Build history of the part. All positions in model axes, mm. Coordinates: 2 decimals unless noted, no trailing zeros. Order: outer loops, then holes, each group sorted by start corner. A loop starts at its lowest first (then second) coordinate and runs counter-clockwise, first axis right, second up. Notation, with made-up numbers: (-35, 22) - (-8, 22) arc R27 ccw to (-8, 54) - close; hole circle Ø10 at (-37.5, 61.25). An arc over 180 degrees is marked (long way). Write each question's results on one line, items separated by ' | '.
from build123d import *

# Parameters (mm, degrees)
SKETCH_1_W          = 38
SKETCH_1_H          = 35
EXTRUDE_1_DEPTH     = 5
CHAMFER_1_SIZE      = 0.5
SKETCH_2_R          = 2.25
SKETCH_2_R_2        = 2
CUT_EXTRUDE_1_DEPTH = 52.903757089


with BuildPart() as part:
    # 草图1 → 凸台-拉伸1 (new body)
    with BuildSketch(Plane(origin=(0, 0, 0), x_dir=(1, 0, 0), z_dir=(0, 1, 0))):
        with Locations((19, 17.5)):
            Rectangle(SKETCH_1_W, SKETCH_1_H)
    extrude(amount=EXTRUDE_1_DEPTH)

    # 倒角1
    chamfer_1_edges = [part.edges().sort_by_distance(p)[0] for p in [
        (38, 5, -17.5),
        (19, 5, -35),
        (0, 5, -17.5),
        (19, 0, -35),
        (38, 0, -17.5),
        (19, 0, 0),
        (0, 0, -17.5),
        (19, 5, 0),
        (0, 2.5, -35),
        (38, 2.5, -35),
        (38, 2.5, 0),
        (0, 2.5, 0),
    ]]
    chamfer(chamfer_1_edges, length=CHAMFER_1_SIZE)

    # 草图2 → 切除-拉伸1 (cut, through all)
    with BuildSketch(Plane.XZ):
        with Locations(Location((5, -5, 0), (0, 0, 270))):
            Circle(SKETCH_2_R)
        with Locations(Location((5, -30, 0), (0, 0, 270))):
            Circle(SKETCH_2_R)
        with Locations(Location((33, -30, 0), (0, 0, 270))):
            Circle(SKETCH_2_R)
        with Locations(Location((33, -5, 0), (0, 0, 270))):
            Circle(SKETCH_2_R)
        with Locations(Location((5, -12, 0), (0, 0, 270))):
            Circle(SKETCH_2_R_2)
        with Locations(Location((5, -23, 0), (0, 0, 270))):
            Circle(SKETCH_2_R_2)
    extrude(amount=-CUT_EXTRUDE_1_DEPTH, mode=Mode.SUBTRACT)


solid = part.part
1. Band-saw the part on D-D on y = 3.9. Give the cut face in (x, z).
Solved:
outline: (0, -34.5) - (0.5, -35) - (37.5, -35) - (38, -34.5) - (38, -0.5) - (37.5, 0) - (0.5, 0) - (0, -0.5) - close; hole circle Ø4.5 at (5, -30); hole circle Ø4.5 at (5, -5); hole circle Ø4 at (5, -23); hole circle Ø4 at (5, -12); hole circle Ø4.5 at (33, -30); hole circle Ø4.5 at (33, -5)
2. Drop a flat-ended pin along its axis: pin 1 Ø2.5 at (x, z) = (5, -12) entering from +Y. Give the stop position or say it passes through.
Solved:
pin 1: passes through
3. Band-saw the part on C-C on z = -30. Give the cut face in (x, y), then the cut area to 4 significant figures.
Solved:
outline: (0, 0.5) - (0.5, 0) - (2.75, 0) - (2.75, 5) - (0.5, 5) - (0, 4.5) - close; (7.25, 0) - (30.75, 0) - (30.75, 5) - (7.25, 5) - close; (35.25, 0) - (37.5, 0) - (38, 0.5) - (38, 4.5) - (37.5, 5) - (35.25, 5) - close | area: 144.5 mm2
4. Two-plate mould, pull along X, no slides. Class faces 1 (the face through (0, 2, -17)), 2 (the face through (5, 2, -21)), 3 (the face through (19, 2, 0)): +X half, -X half, draft (parallel to the pull), parting line (faces both ways), or undercut.
Solved:
face 1: -X half | face 2: undercut | face 3: draft
5. Band-saw the part on B-B on x = 33. Give the cut face in (y, z), then the cut area to 4 significant figures.
Solved:
outline: (0, -34.5) - (0.5, -35) - (4.5, -35) - (5, -34.5) - (5, -32.25) - (0, -32.25) - close; (0, -27.75) - (5, -27.75) - (5, -7.25) - (0, -7.25) - close; (0, -2.75) - (5, -2.75) - (5, -0.5) - (4.5, 0) - (0.5, 0) - (0, -0.5) - close | area: 129.5 mm2
6. Probe line 1 (X direction, y = 0.6, z = -3); line 2 (X direction, y = 1.65, z = -4.5); line 3 (Z direction, x = 6.5, y = 2.1). List the from-to ranges inside material, lowest first.
Solved:
line 1: x = 0 to 3.97, 6.03 to 31.97, 34.03 to 38 | line 2: x = 0 to 2.81, 7.19 to 30.81, 35.19 to 38 | line 3: z = -35 to -31.68, -28.32 to -24.32, -21.68 to -13.32, -10.68 to -6.68, -3.32 to 0
7. Band-saw the part on A-A on z = -23. Give the cut face in (x, y), then the cut area to 4 significant figures.
Solved:
outline: (0, 0.5) - (0.5, 0) - (3, 0) - (3, 5) - (0.5, 5) - (0, 4.5) - close; (7, 0) - (37.5, 0) - (38, 0.5) - (38, 4.5) - (37.5, 5) - (7, 5) - close | area: 169.5 mm2
